Autodesk Inventor part; units mm, degrees
ref_plane "Work Plane1" through (0, 0, 4.5) normal (0, 0, 1) x (1, 0, 0)
ref_plane "YZ Plane" through (0, 0, 0) normal (1, 0, 0) x (0, 1, 0)
ref_plane "XZ Plane" through (0, 0, 0) normal (0, 1, 0) x (-1, 0, 0)
sketch "Sketch1" plane through (0, 0, 0) normal (0, 0, 1) x (1, 0, 0)
  circle A0 centre (0, 0) radius 22.4
  dimension "d0" = 44.8
extrude "Extrusion1" add sketch "Sketch1" along normal blind 11
sketch "Sketch8" plane through (0, 0, 0) normal (0, 0, -1) x (-1, 0, 0)
  circle A0 centre (0, 0) radius 26
  dimension "d23" = 52
extrude "Extrusion7" add sketch "Sketch8" against normal blind 4
sketch "Sketch2" plane through (0, 0, 0) normal (0, 0, -1) x (-1, 0, 0)
  circle A0 centre (19.155, 0) radius 1.75
  circle A1 centre (-9.5775, 16.5887) radius 1.75
  circle A2 centre (-9.5775, -16.5887) radius 1.75
  point P0 (0, 0)
  dimension "d3" = 3.5
  dimension "d4" = 19.155
  dimension "d7" = 360
extrude "Extrusion2" cut sketch "Sketch2" against normal through all
sketch "Sketch3" plane through (0, 0, 11) normal (0, 0, 1) x (1, 0, 0)
  circle A0 centre (0, 0) radius 6
  dimension "d11" = 12
extrude "Extrusion3" cut sketch "Sketch3" against normal blind 2
sketch "Sketch4" plane through (0, 0, 11) normal (0, 0, 1) x (1, 0, 0)
  circle A0 centre (0, 0) radius 6
  line L0 (11.547, 0) -> (5.7735, -10)
  line L1 (5.7735, -10) -> (-5.7735, -10)
  line L2 (-5.7735, -10) -> (-11.547, 0)
  line L3 (-11.547, 0) -> (-5.7735, 10)
  line L4 (-5.7735, 10) -> (5.7735, 10)
  line L5 (5.7735, 10) -> (11.547, 0)
  circle A1 centre (0, 0) radius 6
  dimension "d14" = 10
extrude "Extrusion4" cut sketch "Sketch4" against normal blind 1.5
sketch "Sketch5" plane through (0, 0, 0) normal (0, 0, -1) x (-1, 0, 0)
  line L0 (5.7735, 10) -> (-5.7735, 10)
  line L1 (-5.7735, 10) -> (5.7735, 10)
  line L2 (5.7735, 10) -> (11.547, 0)
  line L3 (11.547, 0) -> (5.7735, -10)
  line L4 (5.7735, -10) -> (-5.7735, -10)
  line L5 (-5.7735, -10) -> (-11.547, 0)
  line L6 (-11.547, 0) -> (-5.7735, 10)
  point P0 (0, 0)
  point P1 (0, 0)
extrude "Extrusion5" add sketch "Sketch5" along normal blind 1.5
ref_plane "Work Plane1" through (0, 0, 4.5) normal (0, 0, 1) x (1, 0, 0)
sketch "Sketch6" plane through (0, 0, 4.5) normal (0, 0, 1) x (1, 0, 0)
  circle A0 centre (0, 0) radius 22.6071
  circle A1 centre (0, 0) radius 21.1
  dimension "d20" = 42.2
extrude "Extrusion6" [suppressed]
sketch "Sketch7" plane through (0, 0, 0) normal (0, 0, -1) x (-1, 0, 0)
  point P0 (0, 0)
sketch "Sketch9" plane through (0, 0, 9.5) normal (0, 0, 1) x (1, 0, 0)
  circle A0 centre (0, 0) radius 6
  circle A1 centre (0, 0) radius 8.1
  dimension "d26" = 16.2
extrude "Extrusion8" cut sketch "Sketch9" against normal blind 3 contours A0 | A1
sketch "Sketch10" plane through (0, 0, 6.5) normal (0, 0, 1) x (1, 0, 0)
  circle A0 centre (0, 0) radius 6
  dimension "d29" = 12
extrude "Extrusion9" cut sketch "Sketch10" against normal through all
properties part number "Planet Carrier 2"
Could you check a few things on this model? Use its own coordinates, in mm. A direction names the side the tool comes from. Round coordinates to 2 decimals unless told otherwise and drop trailing zeros. Order: outer loops, then holes, each group sorted by start corner. A loop starts at its lowest first (then second) coordinate and runs counter-clockwise, first axis right, second up.
Q1. Imagine slicing it at B-B, the plane y = 3.5. List the corners of the cut face in (x, z) for me.
Geometry says:
outline: (-25.76, 0) - (-9.53, 0) - (-9.53, -1.5) - (-4.87, -1.5) - (-4.87, 6.5) - (-7.3, 6.5) - (-7.3, 9.5) - (-9.53, 9.5) - (-9.53, 11) - (-22.12, 11) - (-22.12, 4) - (-25.76, 4) - close; (4.87, -1.5) - (9.53, -1.5) - (9.53, 0) - (25.76, 0) - (25.76, 4) - (22.12, 4) - (22.12, 11) - (9.53, 11) - (9.53, 9.5) - (7.3, 9.5) - (7.3, 6.5) - (4.87, 6.5) - close
Q2. Imagine slicing it at C-C, the plane x = 10.5. List the corners of the cut face in (y, z) for me.
Geometry says:
outline: (-23.79, 0) - (-18.08, 0) - (-18.08, 11) - (-19.79, 11) - (-19.79, 4) - (-23.79, 4) - close; (-15.1, 0) - (-1.81, 0) - (-1.81, -1.5) - (1.81, -1.5) - (1.81, 0) - (15.1, 0) - (15.1, 11) - (1.81, 11) - (1.81, 9.5) - (-1.81, 9.5) - (-1.81, 11) - (-15.1, 11) - close; (18.08, 0) - (23.79, 0) - (23.79, 4) - (19.79, 4) - (19.79, 11) - (18.08, 11) - close
Q3. Which directions (+Z, -Z, +X, -X, +Y, -Y) give clear straight access to the entire face, cutting with the end or side of a thin tool? Please do faces 4 (the face through (0, 10, 10)), 5 (the face through (-6, 0, 3)), 6 (the face through (10, -5, 11)), 7 (the face through (0, -11, 0)), 8 (the face through (-8.62, 5.07, -0.74)).
Geometry says:
face 4: +Z
face 5: +Z, -Z
face 6: +Z, +X, -X, +Y, -Y
face 7: -Z
face 8: -Z, -X, +Y
Q4. I'm going to push flat-ended pins straight in: P1, Ø10, axis at x = -7, y = 17.5, coming from the -Z side; P2, Ø1.5, axis at y = 2.5, z = 0, coming from the -X side; P3, Ø1.6, axis at x = 0, z = 10.5, coming from the -Y side; P4, Ø3, axis at x = -19.155, y = 0, coming from the +Z side. Where does each tip first touch, or does it pass through?
Geometry says:
P1: stops at z = 0
P2: stops at x = -25.94
P3: stops at y = -22.4
P4: passes through
Q5. Imagine slicing it at A-A, the plane x = 0. List the corners of the cut face in (y, z) for me.
Geometry says:
outline: (-26, 0) - (-10, 0) - (-10, -1.5) - (-6, -1.5) - (-6, 6.5) - (-8.1, 6.5) - (-8.1, 9.5) - (-10, 9.5) - (-10, 11) - (-22.4, 11) - (-22.4, 4) - (-26, 4) - close; (6, -1.5) - (10, -1.5) - (10, 0) - (26, 0) - (26, 4) - (22.4, 4) - (22.4, 11) - (10, 11) - (10, 9.5) - (8.1, 9.5) - (8.1, 6.5) - (6, 6.5) - close
Q6. Please list where these lines run through material, in increasing order: probe 1 along Y at (x, z) = (0, 3.75); probe 2 along Y at (x, z) = (9, 1); probe 3 along Y at (x, z) = (0, 8.5).
Geometry says:
probe 1: y = -26 to -6, 6 to 26
probe 2: y = -24.39 to -18.24, -14.94 to 14.94, 18.24 to 24.39
probe 3: y = -22.4 to -8.1, 8.1 to 22.4
Q7. Thinking about a two-plate mould opening in Y: for faces 1 (the face through (0, -10, -1)), 2 (the face through (8.7, 4.93, -0.74)), 3 (the face through (8.7, -4.93, 10.26)), which applies, released by +Y, released by -Y, zero draft, split by the parting line, or undercut?
Geometry says:
face 1: released by -Y
face 2: released by +Y
face 3: undercut
Q8. Imagine slicing it at D-D, the plane z = 5. State how many separate pieces and enclosed holes the cut face has, then the cut area to 3 significant figures.
Geometry says:
separate pieces: 1
enclosed holes: 4
area: 1,430 mm2
